Build history of the part. All positions in model axes, mm. Coordinates: 2 decimals unless noted, no trailing zeros. Loops run counter-clockwise (first coordinate to the right, second up) from the corner with the lowest first, then second, coordinate; pieces in that order, holes last.
Item 1: Cut at C-C (z = 15). List the corners of the cut face in (x, y), and give its area (3 significant figures).
Item 2: Drill centre lines: line 1 along Z through (x, y) = (147, -19.5); line 2 along Z through (x, y) = (190, -6.25); line 3 along Y through (x, z) = (28, 110.5). Where is each one in solid material? Low to high.
Item 3: Cut at A-A (y = -10.75). List the corners of the cut face in (x, z).
Item 4: Mould opens along Z. For faces 1 (the face through (187, -10, 130)), 2 (the face through (197, 0, 66)), 3 (the face through (187, -10, 0)), 4 (the face through (190, -15.9, 112)) say: released by +Z, released by -Z, zero draft, split by the parting line, or undercut.
Item 5: Cut at B-B (x = 61.5). List the corners of the cut face in (y, z), and give its area (3 significant figures).
Item 6: Flat gauge pins, fed straight in: pin 1 (6 mm diameter, centred on x = 321.5, z = 104, fed in from -Y); pin 2 (1.5 mm diameter, centred on y = -18.5, z = 110.5, fed in from +X); pin 3 (6 mm diameter, centred on y = -11, z = 22.5, fed in from -X); pin 4 (1 mm diameter, centred on y = -9, z = 83.5, fed in from -X). Where does each tip first touch, or does it go through?
from build123d import *

# Parameters (mm, degrees)
F0_W     = 380
F0_H     = 130
F1_DEPTH = 21
F2_W     = 375
F2_H     = 17
F3_DEPTH = 5.1
F4_SIZE  = 20
F6_D     = 5


with BuildPart() as f1:
    # F0 (on Front) → F1 (new body)
    with BuildSketch(Plane.XZ):
        with Locations((190, 65)):
            Rectangle(F0_W, F0_H)
    extrude(amount=F1_DEPTH)

    # F2 (on face) → F3 (cut, symmetric)
    with BuildSketch(Plane.XZ.offset(21)):
        with Locations((192.5, 111.5)):
            Rectangle(F2_W, F2_H)
    extrude(amount=F3_DEPTH, both=True, mode=Mode.SUBTRACT)

    # F4
    f4_edges = [f1.edges().sort_by_distance(p)[0] for p in [
        (0, 0, 65),
    ]]
    chamfer(f4_edges, length=F4_SIZE)

    # F6 (through all)
    with Locations(Plane.XZ.offset(21)):
        with Locations((190, 65)):
            Hole(F6_D / 2)


solid = f1.part
Filled sheet:
1. outline: (0, -21) - (380, -21) - (380, 0) - (20, 0) - (0, -20) - close
1. area: 7,780 mm2
2. line 1: z = 0 to 103, 120 to 130
2. line 2: z = 0 to 62.5, 67.5 to 130
2. line 3: y = -15.9 to 0
3. outline: (9.25, 0) - (380, 0) - (380, 130) - (9.25, 130) - close; hole circle Ø5 at (190, 65)
4. face 1: released by +Z
4. face 2: zero draft
4. face 3: released by -Z
4. face 4: undercut
5. outline: (-21, 0) - (0, 0) - (0, 130) - (-21, 130) - (-21, 120) - (-15.9, 120) - (-15.9, 103) - (-21, 103) - close
5. area: 2,640 mm2
6. pin 1: stops at y = -21
6. pin 2: stops at x = 5
6. pin 3: stops at x = 6
6. pin 4: stops at x = 10.5
